Geometry: see drawing. Coordinates: mm, zero at the bounding-box minimum. A direction names the side the tool comes from. Give positions to 0.01 mm unless a question says otherwise; leave off trailing zeros. Order: outer loops, then holes, each group sorted by start corner. A loop starts at its lowest first (then second) coordinate and runs counter-clockwise, first axis right, second up. Notation, with made-up numbers: (-38.75, 37.5) - (-30.75, 37.5) arc R16 cw to (-30.75, 49.5) - close; hole circle Ø10 at (-15, 8.5). An arc over 180 degrees is marked (long way). One line per item, written item: value.
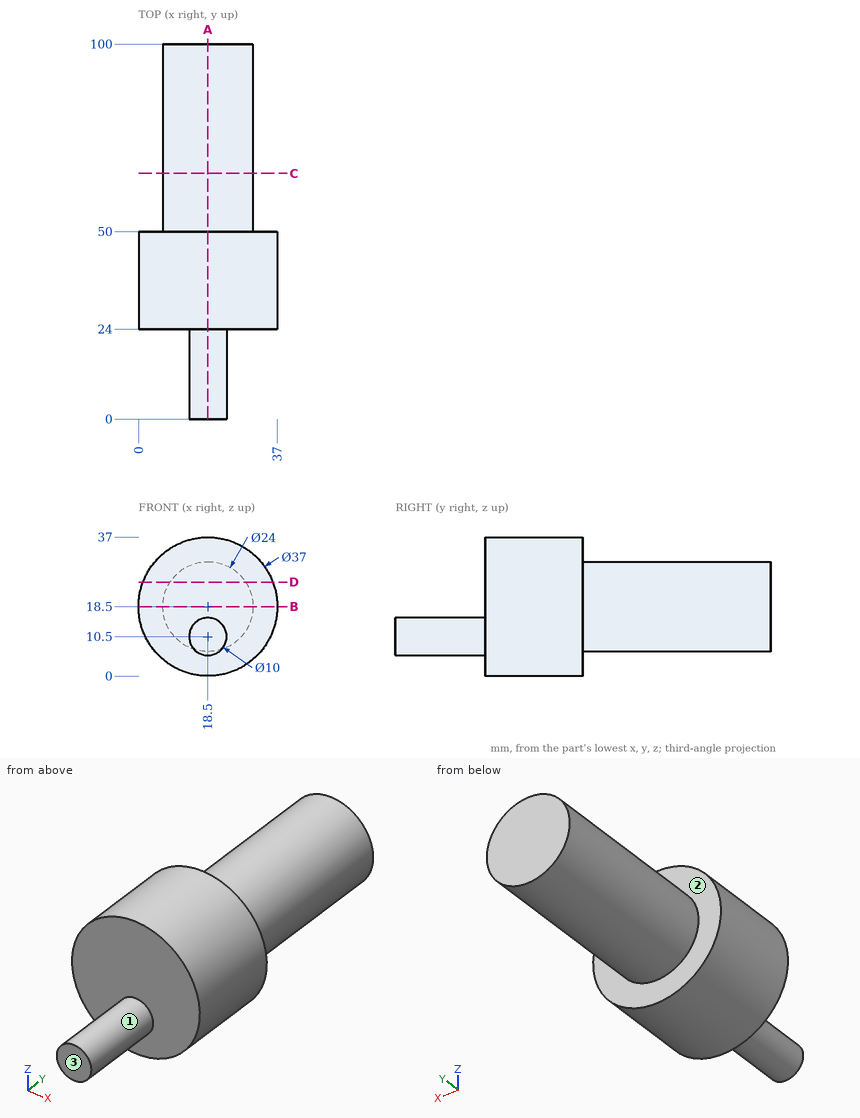
1) First-contact query: pin 1 (5 mm diameter, centred on x = 16, y = 75, fed in from -Z); pin 2 (12 mm diameter, centred on x = 33, z = 5.5, fed in from -Y); pin 3 (4 mm diameter, centred on y = 70, z = 21, fed in from -X). Flat tips, straight axial feed; report the tip coordinate or a pass-through.
Answers below:
pin 1: z = 6.5
pin 2: y = 24
pin 3: x = 6.51
2) Section D-D, the plane z = 25. Return loops of the section in (x, y), then the cut area to 3 significant figures.
Answers below:
outline: (1.18, 24) - (35.82, 24) - (35.82, 50) - (28.59, 50) - (28.59, 100) - (8.41, 100) - (8.41, 50) - (1.18, 50) - close
area: 1,910 mm^2
3) Section C-C, the plane y = 65.5. Return loops of the section in (x, z), then the cut area to 3 significant figures.
Answers below:
outline: circle Ø24 at (18.5, 18.5)
area: 452 mm^2
4) Section B-B, the plane z = 18.5. Return loops of the section in (x, y), then the cut area to 3 significant figures.
Answers below:
outline: (0, 24) - (37, 24) - (37, 50) - (30.5, 50) - (30.5, 100) - (6.5, 100) - (6.5, 50) - (0, 50) - close
area: 2,160 mm^2
5) Material intervals for line 1 along Y through (x, z) = (14.5, 16.5); line 2 along X through (y, z) = (65, 18.5); line 3 along Y through (x, z) = (34, 24), sorted ascending.
Answers below:
line 1: 24 to 100
line 2: 6.5 to 30.5
line 3: 24 to 50
6) Set-up query: the marked faces 1, 2 and 3. Return all of +Z, -Z, +X, -X, +Y, -Y with unobstructed straight access to the full face (end or side cutting, diameter ignored); none if empty.
Answers below:
face 1: -Y
face 2: +Y
face 3: +Z, -Z, +X, -X, -Y
7) Section A-A, the plane x = 18.5. Return loops of the section in (y, z), then the cut area to 3 significant figures.
Answers below:
outline: (0, 5.5) - (24, 5.5) - (24, 0) - (50, 0) - (50, 6.5) - (100, 6.5) - (100, 30.5) - (50, 30.5) - (50, 37) - (24, 37) - (24, 15.5) - (0, 15.5) - close
area: 2,400 mm^2
